For this review, take the finished solid that the model builds, in its own axes (mm). Face numbers are marked on the shaded views. Round coordinates to 2 decimals unless told otherwise and drop trailing zeros. Loops run counter-clockwise (first coordinate to the right, second up) from the corner with the lowest first, then second, coordinate; pieces in that order, holes last.
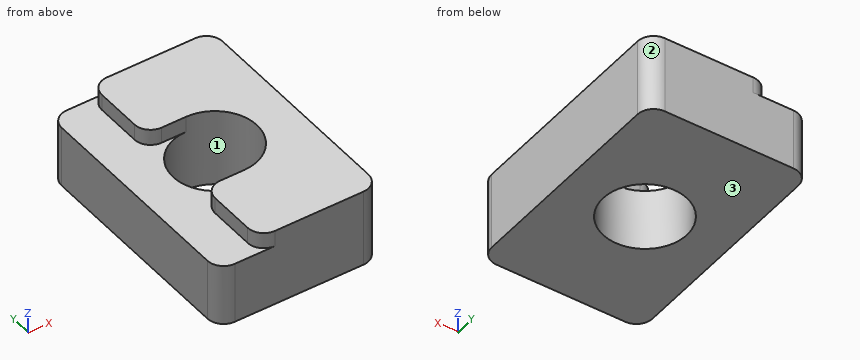
```python
from build123d import *

# Parameters (mm, degrees)
F0_R     = 2.6
F1_DEPTH = 4.83
F3_DEPTH = 1
F4_R     = 1


with BuildPart() as f1:
    # F0 (on Top) → F1 (new body)
    with BuildSketch(Plane.XY):
        with BuildLine():
            Line((-4, -7.5), (4, -7.5))
            ThreePointArc((4, -7.5), (4.7071067812, -7.2071067812), (5, -6.5))
            Line((5, -6.5), (5, 6.5))
            ThreePointArc((5, 6.5), (4.7071067812, 7.2071067812), (4, 7.5))
            Line((4, 7.5), (-4, 7.5))
            ThreePointArc((-4, 7.5), (-4.7071067812, 7.2071067812), (-5, 6.5))
            Line((-5, 6.5), (-5, -6.5))
            ThreePointArc((-5, -6.5), (-4.7071067812, -7.2071067812), (-4, -7.5))
        make_face()
        Circle(F0_R, mode=Mode.SUBTRACT)
    extrude(amount=F1_DEPTH)

    # F2 (on face) → F3 (cut)
    with BuildSketch(Plane.XY.offset(4.83)):
        with BuildLine():
            Line((-2.5, 2.6), (-2.5, 7.5))
            Line((-2.5, 7.5), (-4, 7.5))
            ThreePointArc((-4, 7.5), (-4.7071067812, 7.2071067812), (-5, 6.5))
            Line((-5, 6.5), (-5, -6.5))
            ThreePointArc((-5, -6.5), (-4.7071067812, -7.2071067812), (-4, -7.5))
            Line((-4, -7.5), (-2.5, -7.5))
            Line((-2.5, -7.5), (-2.5, -2.6))
            Line((-2.5, -2.6), (0, -2.6))
            ThreePointArc((0, -2.6), (-2.6, 0), (0, 2.6))
            Line((0, 2.6), (-2.5, 2.6))
        make_face()
    extrude(amount=-F3_DEPTH, mode=Mode.SUBTRACT)

    # F4
    f4_edges = [f1.edges().sort_by_distance(p)[0] for p in [
        (-2.5, -7.5, 4.33),
        (-2.5, 2.6, 4.33),
        (-2.5, -2.6, 4.33),
        (-2.5, 7.5, 4.33),
    ]]
    fillet(f4_edges, radius=F4_R)


solid = f1.part
```
(1) Insertion check: pin 1 Ø4 at (x, y) = (0, 0) entering from +Z; pin 2 Ø0.5 at (y, z) = (-5, 4.5) entering from -X. Each pin has a flat end and moves straight along its axis. Give the tip position at first contact, or say it passes through.
(2) For L1, parallel to Y at x = 0, z = 1.7; L2, parallel to X at y = 0, z = 1.45; L3, parallel to Z at x = -3.75, y = 2.75, list the stretches that pass through material, from the lowest coordinate up.
(3) Add section C-C (x = -0.75). Give the boundary of the cut face in (y, z), plus the area to 3 significant figures.
(4) Add section B-B (z = 1.75). Give the boundary of the cut face in (x, y), plus the area to 3 significant figures.
(5) Add section D-D (x = 0.25). Give the boundary of the cut face in (y, z), plus the area to 3 significant figures.
(6) The part is to be moulded in two halves that separate along X. For the marked faces 1, 2 and 3, say which applies: pulls with the +X half, pulls with the -X half, needs draft (parallel to the pull), parting line crosses it, or undercut.
(7) Add section A-A (y = 0). Give the boundary of the cut face in (x, z), plus the area to 3 significant figures.
Outcome:
1. pin 1: passes through
1. pin 2: stops at x = -2.5
2. L1: y = -7.5 to -2.6, 2.6 to 7.5
2. L2: x = -5 to -2.6, 2.6 to 5
2. L3: z = 0 to 3.83
3. outline: (-7.5, 0) - (-2.49, 0) - (-2.49, 3.83) - (-2.6, 3.83) - (-2.6, 4.83) - (-7.5, 4.83) - close; (2.49, 0) - (7.5, 0) - (7.5, 4.83) - (2.6, 4.83) - (2.6, 3.83) - (2.49, 3.83) - close
3. area: 48.2 mm2
4. outline: (-5, -6.5) arc R1 ccw to (-4, -7.5) - (4, -7.5) arc R1 ccw to (5, -6.5) - (5, 6.5) arc R1 ccw to (4, 7.5) - (-4, 7.5) arc R1 ccw to (-5, 6.5) - close; hole circle Ø5.2 at (0, 0)
4. area: 128 mm2
5. outline: (-7.5, 0) - (-2.59, 0) - (-2.59, 4.83) - (-7.5, 4.83) - close; (2.59, 0) - (7.5, 0) - (7.5, 4.83) - (2.59, 4.83) - close
5. area: 47.5 mm2
6. face 1: undercut
6. face 2: pulls with the +X half
6. face 3: needs draft
7. outline: (-5, 0) - (-2.6, 0) - (-2.6, 3.83) - (-5, 3.83) - close; (2.6, 0) - (5, 0) - (5, 4.83) - (2.6, 4.83) - close
7. area: 20.8 mm2
